Can you work these out from the model? Positions are in its coordinate system, mm. Face numbers are marked on the shaded views. A direction names the side the tool comes from. Give positions to 0.01 mm unless a question says otherwise; leave off trailing zeros. Write each loop counter-clockwise with the first axis right and the second up, starting at its lowest first coordinate (ties: lowest second). Pieces come first, ordered by that corner, then holes. Notation, with made-up numbers: (-2, 68) -> (50, 68) arc R13 cw to (50, 73) -> close; hole circle Ø2 at (-35, 32). An arc over 180 degrees is marked (long way). One line per item, written item: value.
from build123d import *

# Parameters (mm, degrees)
SKETCH1_R            = 34
SKETCH1_R_2          = 31.25
BOSS_EXTRUDE1_DEPTH  = 25.5
SKETCH2_R            = 34
BOSS_EXTRUDE2_DEPTH  = 3
SKETCH5_R            = 3.5
CUT_EXTRUDE3_DEPTH   = 51
BOSS_EXTRUDE9_START  = 25.5
BOSS_EXTRUDE9_DEPTH  = 28.5
CUT_SWEEP6_PROFILE_R = 11
SKETCH219_R          = 12
CUT_EXTRUDE10_DEPTH  = 20
SKETCH227_W          = 22
SKETCH227_H          = 10.782706647
SKETCH227_R          = 1.55
BOSS_EXTRUDE11_DEPTH = 4
FILLET1_R            = 3
FILLET2_R            = 3


with BuildPart() as part:
    # Sketch1 → Boss-Extrude1 (new body)
    with BuildSketch(Plane.XY):
        Circle(SKETCH1_R)
        Circle(SKETCH1_R_2, mode=Mode.SUBTRACT)
    extrude(amount=BOSS_EXTRUDE1_DEPTH)

    # Sketch2 → Boss-Extrude2 (add)
    with BuildSketch(Plane.XY.offset(25.5)):
        Circle(SKETCH2_R)
    extrude(amount=BOSS_EXTRUDE2_DEPTH)

    # Sketch5 → Cut-Extrude3 (cut)
    with BuildSketch(Plane.XY.offset(28.5)):
        Circle(SKETCH5_R)
    extrude(amount=-CUT_EXTRUDE3_DEPTH, mode=Mode.SUBTRACT)

    # Sketch3 → Boss-Extrude9 (add)
    with BuildSketch(Plane(origin=(0, 0, 25.5), x_dir=(-1, 0, 0), z_dir=(0, 0, -1)).offset(BOSS_EXTRUDE9_START)):
        with BuildLine():
            Line((24.25, -50), (50.25, -50))
            Line((50.25, -50), (50.25, -21.368098989))
            ThreePointArc((50.25, -21.368098989), (35.814519651, 16.017355688), (0, 34))
            Line((0, 34), (0, 31.25))
            ThreePointArc((0, 31.25), (28.21801379, 13.427814332), (24.25, -19.710403344))
            Line((24.25, -19.710403344), (24.25, -50))
        make_face()
    extrude(amount=-BOSS_EXTRUDE9_DEPTH)

    # Cut-Sweep6: sweep along a path in Sketch28
    with BuildLine(Plane(origin=(0, 0, 14.25), x_dir=(-1, 0, 0), z_dir=(0, 0, -1))) as cut_sweep6_path:
        Line((37.25, -50), (37.25, -21.368098989))
        ThreePointArc((37.25, -21.368098989), (28.563956157, 4.353039323), (6.0625, 19.54214017))
    # Cut-Sweep6 profile (on start of the path) → Cut-Sweep6 (sweep, cut)
    with BuildSketch(Plane(origin=(-37.25, -50, 14.25), x_dir=(0, 0, 1), z_dir=(0, 1, 0))):
        Circle(CUT_SWEEP6_PROFILE_R)
    sweep(path=cut_sweep6_path.line, mode=Mode.SUBTRACT)

    # Sketch219 → Cut-Extrude10 (cut)
    with BuildSketch(Plane.XZ.offset(50)):
        with Locations(Location((-37.25, 14.25, 0), (0, 0, 270))):
            Circle(SKETCH219_R)
    extrude(amount=-CUT_EXTRUDE10_DEPTH, mode=Mode.SUBTRACT)

    # Sketch227 → Boss-Extrude11 (add)
    # profile 1 of 2: a face of its own
    with BuildSketch(Plane.XY.offset(28.5)):
        with Locations((0, 30.358646677)):
            Rectangle(SKETCH227_W, SKETCH227_H)
        with Locations((-6, 30.25)):
            Circle(SKETCH227_R, mode=Mode.SUBTRACT)
        with Locations((6, 30.25)):
            Circle(SKETCH227_R, mode=Mode.SUBTRACT)
    # profile 2 of 2: a face of its own
    with BuildSketch(Plane.XY.offset(28.5)):
        with Locations((0, -30.358646677)):
            Rectangle(SKETCH227_W, SKETCH227_H)
        with Locations((-6, -30.25)):
            Circle(SKETCH227_R, mode=Mode.SUBTRACT)
        with Locations((6, -30.25)):
            Circle(SKETCH227_R, mode=Mode.SUBTRACT)
    extrude(amount=BOSS_EXTRUDE11_DEPTH)

    # Fillet1
    # the kernel refuses this fillet: 3 mm, written as the material it takes off along each edge
    with BuildSketch(Plane(origin=(-18.5, 35.75, 28.5), x_dir=(0, -1, 0), z_dir=(1, 0, 0))) as fillet1_piece_1_section:
        with BuildLine():
            CenterArc((FILLET1_R, -FILLET1_R), FILLET1_R, 90, 90)
            Line((0, -FILLET1_R), (0, 0))
            Line((0, 0), (FILLET1_R, 0))
        make_face()
    fillet1_piece_1 = extrude(amount=37, mode=Mode.PRIVATE)
    fillet1_piece_1 = fillet1_piece_1 - Plane(origin=(0, 0, 29.19390081), x_dir=(1, 0, 0), z_dir=(0, 0, -1)) * Cylinder(34, 86, mode=Mode.PRIVATE)
    add(fillet1_piece_1, mode=Mode.SUBTRACT)

    # Fillet2
    # the kernel refuses this fillet: 3 mm, written as the material it takes off along each edge
    with BuildSketch(Plane(origin=(-18.5, -35.75, 28.5), x_dir=(0, 1, 0), z_dir=(1, 0, 0))) as fillet2_piece_1_section:
        with BuildLine():
            CenterArc((FILLET2_R, FILLET2_R), FILLET2_R, 180, 90)
            Line((0, FILLET2_R), (0, 0))
            Line((0, 0), (FILLET2_R, 0))
        make_face()
    fillet2_piece_1 = extrude(amount=37, mode=Mode.PRIVATE)
    fillet2_piece_1 = fillet2_piece_1 - Plane(origin=(0, 0, 29.19390081), x_dir=(1, 0, 0), z_dir=(0, 0, -1)) * Cylinder(34, 86, mode=Mode.PRIVATE)
    add(fillet2_piece_1, mode=Mode.SUBTRACT)


solid = part.part
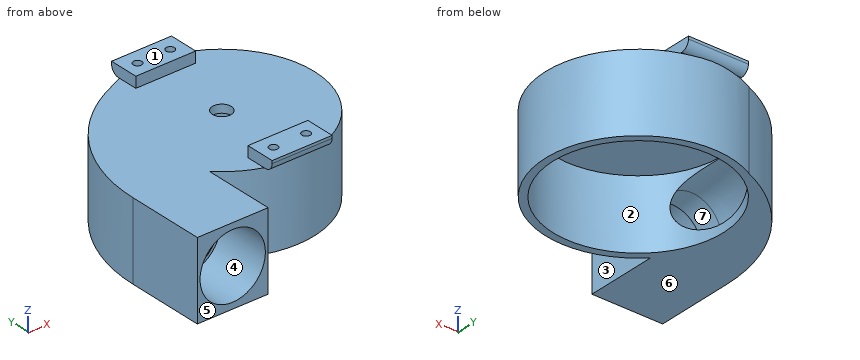
1) If we section it at D-D (z = 6.5): Write out the boundary of the cut face in (x, y), and give its area (3 significant figures).
Answer list:
outline: (-50.25, -50) -> (-46.41, -50) -> (-46.41, -30) -> (-45.06, -30) -> (-45.06, -21.37) arc R50.23 cw to (-24.93, 18.84) arc R31.25 cw (long way) to (-28.42, -13) arc R34.62 ccw to (-29.44, -21.37) -> (-29.44, -30) -> (-28.09, -30) -> (-28.09, -50) -> (-24.25, -50) -> (-24.25, -23.83) arc R34 ccw (long way) to (-16.1, 29.95) arc R55.63 ccw to (-50.25, -21.37) -> close
area: 978 mm^2
2) If we section it at C-C (x = 28.5): Write out the boundary of the cut face in (y, z).
Answer list:
outline: (-18.54, 0) -> (-12.82, 0) -> (-12.82, 25.5) -> (12.82, 25.5) -> (12.82, 0) -> (18.54, 0) -> (18.54, 28.5) -> (-18.54, 28.5) -> close
3) If we section it at B-B (z = 14.25): Write out the boundary of the cut face in (x, y).
Answer list:
outline: (-50.25, -50) -> (-49.25, -50) -> (-49.25, -30) -> (-48.25, -30) -> (-48.25, -21.37) arc R53.43 cw to (-8.98, 30.15) -> (-8.92, 29.95) arc R31.25 cw (long way) to (-25.99, -17.35) arc R31.43 ccw to (-26.25, -21.37) -> (-26.25, -30) -> (-25.25, -30) -> (-25.25, -50) -> (-24.25, -50) -> (-24.25, -23.83) arc R34 ccw (long way) to (-16.1, 29.95) arc R55.63 ccw to (-50.25, -21.37) -> close
4) If we section it at A-A (x = 0): Write out the boundary of the cut face in (y, z), and give its area (3 significant figures).
Answer list:
outline: (-35.75, 31.5) arc R3 ccw to (-34, 28.77) -> (-34, 0) -> (-31.25, 0) -> (-31.25, 25.5) -> (-3.5, 25.5) -> (-3.5, 28.5) -> (-24.97, 28.5) -> (-24.97, 32.5) -> (-35.75, 32.5) -> close; (3.5, 25.5) -> (31.25, 25.5) -> (31.25, 0) -> (34, 0) -> (34, 28.77) arc R3 ccw to (35.75, 31.5) -> (35.75, 32.5) -> (24.97, 32.5) -> (24.97, 28.5) -> (3.5, 28.5) -> close
area: 406 mm^2
5) We'd pull the mould along Z, two halves only. Please class the marked faces 4, 5, 6 and 7: released by +Z, released by -Z, zero draft, split by the parting line, or undercut.
Answer list:
face 4: undercut
face 5: zero draft
face 6: released by -Z
face 7: undercut
6) For the marked faces 1, 2 and 3, which set-ups out of +Z, -Z, +X, -X, +Y, -Y let a thin tool reach every point of the face, with its end or its side?
Answer list:
face 1: +Z, +X, -X, +Y, -Y
face 2: -Z
face 3: +Z, -Z, -Y
7) I need wall thicknesses on L1, parallel to X at y = -30, z = 29; L2, parallel to Y at x = -6, z = 31.25; L3, parallel to Y at x = 0, z = 17. Which ranges of each line are inside material? Lowest first, please.
Answer list:
L1: x = -11 to -7.53, -4.47 to 4.47, 7.53 to 11
L2: y = -35.74 to -31.8, -28.7 to -24.97, 24.97 to 28.7, 31.8 to 35.74
L3: y = -34 to -31.25, 31.25 to 34
8) Will these pins go through, and if not, where does the flat tip stop? pin 1 (10 mm diameter, centred on y = 25.5, z = 29, fed in from +X); pin 2 (9 mm diameter, centred on x = 0, y = 0, fed in from -Z); pin 3 (1.5 mm diameter, centred on y = 1.5, z = 23.5, fed in from -X).
Answer list:
pin 1: stops at x = 27.11
pin 2: stops at z = 25.5
pin 3: stops at x = -45.66
